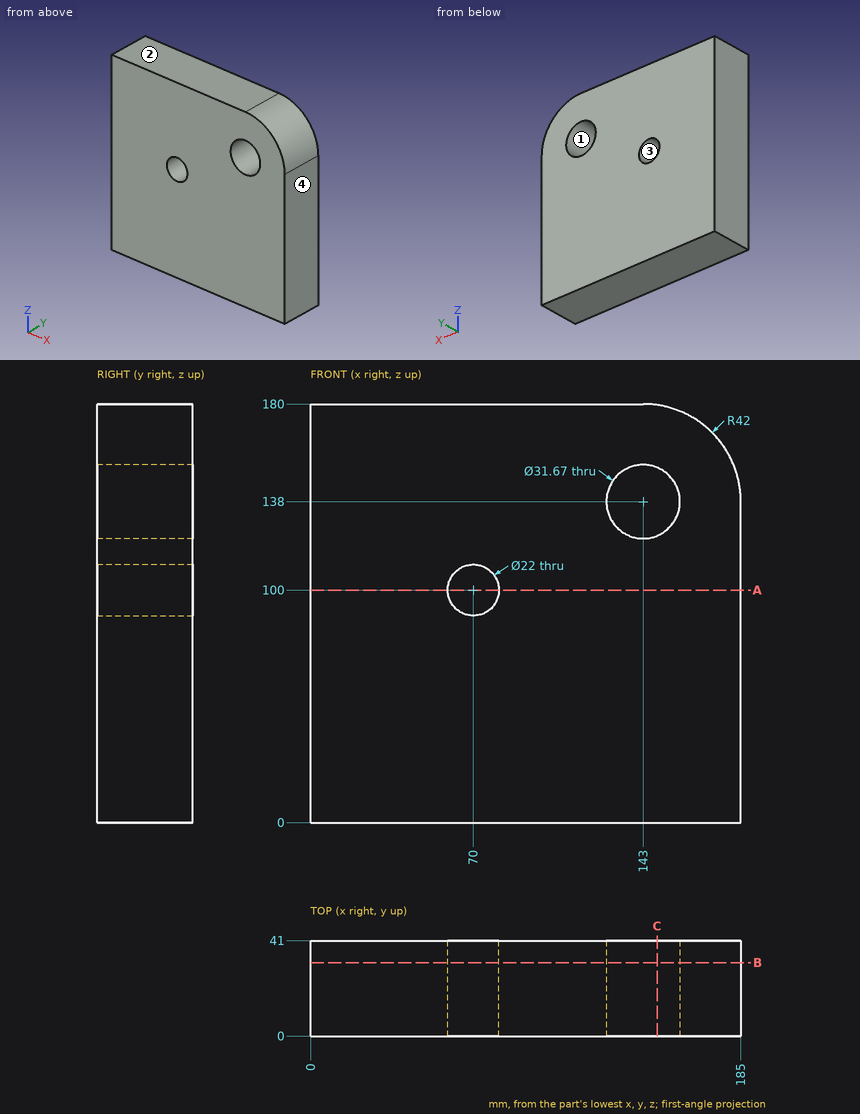
Job drawing, mm, ordinate dimensions from the low corner. One solid piece. Give positions to 0.01 mm unless a question says otherwise; leave off trailing zeros. Order: outer loops, then holes, each group sorted by start corner. A loop starts at its lowest first (then second) coordinate and runs counter-clockwise, first axis right, second up. Notation, with made-up numbers: M 3,74 L 23,74 A31 cw 23,100 Z; hole C 85.5,-24.5 d4. An arc over 180 degrees is marked long. Return JSON: item names as keys, results as strings.
Q1. Flat gauge pins, fed straight in: pin 1 (20 mm diameter, centred on x = 70, z = 100, fed in from +Y); pin 2 (5 mm diameter, centred on y = 17.5, z = 162, fed in from +X). Where does each tip first touch, or does it go through?
Answer list:
{"pin 1": "passes through", "pin 2": "stops at x = 179.08"}
Q2. Band-saw the part on B-B (y = 31.5). Give the cut face in (x, z) (3 decimals), then the cut area to 3 significant figures.
Answer list:
{"outline": "M 0,0 L 185,0 L 185,138 A42 ccw 143,180 L 0,180 Z; hole C 70,100 d22; hole C 143,138 d31.67", "area": "31,800 mm^2"}
Q3. Band-saw the part on A-A (z = 100). Give the cut face in (x, y), then the cut area to 3 significant figures.
Answer list:
{"outline": "M 0,0 L 59,0 L 59,41 L 0,41 Z; M 81,0 L 185,0 L 185,41 L 81,41 Z", "area": "6,680 mm^2"}
Q4. Two-plate mould, pull along X, no slides. Class the marked faces 1, 2, 3 and 4: pulls with the +X half, pulls with the -X half, needs draft (parallel to the pull), parting line crosses it, or undercut.
Answer list:
{"face 1": "undercut", "face 2": "needs draft", "face 3": "undercut", "face 4": "pulls with the +X half"}
Q5. Wall check: probe 1 along X at (y, z) = (22, 100); probe 2 along Z at (x, y) = (70, 20); probe 3 along X at (y, z) = (15.5, 138) (3 decimals). Give the ranges that are in metal, low to high. Write a range as from..to.
Answer list:
{"probe 1": "x = 0..59, 81..185", "probe 2": "z = 0..89, 111..180", "probe 3": "x = 0..127.165, 158.835..185"}
Q6. Band-saw the part on C-C (x = 149). Give the cut face in (y, z), then the cut area to 3 significant figures.
Answer list:
{"outline": "M 0,0 L 41,0 L 41,123.35 L 0,123.35 Z; M 0,152.65 L 41,152.65 L 41,179.57 L 0,179.57 Z", "area": "6,160 mm^2"}
